Geometry check sheet. Reference: the model listing, model coordinates, mm. A direction names the side the tool comes from. Round coordinates to 2 decimals unless told otherwise and drop trailing zeros. Order: outer loops, then holes, each group sorted by start corner. A loop starts at its lowest first (then second) coordinate and runs counter-clockwise, first axis right, second up.
```python
from build123d import *

# Parameters (mm, degrees)
SKETCH2_W           = 127
SKETCH2_H           = 127
SKETCH2_W_2         = 114.3
SKETCH2_H_2         = 114.3
BOSS_EXTRUDE2_DEPTH = 127
CUT_EXTRUDE1_REACH  = 129
CUT_EXTRUDE2_REACH  = 129


with BuildPart() as part:
    # Sketch2 → Boss-Extrude2 (new body)
    with BuildSketch(Plane(origin=(0, 0, 0), x_dir=(1, 0, 0), z_dir=(0, 1, 0))):
        Rectangle(SKETCH2_W, SKETCH2_H)
        Rectangle(SKETCH2_W_2, SKETCH2_H_2, mode=Mode.SUBTRACT)
    extrude(amount=BOSS_EXTRUDE2_DEPTH)

    # Sketch6 → Cut-Extrude1 (cut, up to next)
    with BuildSketch(Plane.ZY.offset(63.5), mode=Mode.PRIVATE) as cut_extrude1_sk1:
        with BuildLine():
            Line((-4.523172318, 109.1946), (-10.873172318, 109.1946))
            ThreePointArc((-10.873172318, 109.1946), (-13.425872318, 111.7473), (-10.873172318, 114.3))
            Line((-10.873172318, 114.3), (-4.523172318, 114.3))
            ThreePointArc((-4.523172318, 114.3), (-1.970472318, 111.7473), (-4.523172318, 109.1946))
        make_face()
    cut_extrude1_tool1 = extrude(cut_extrude1_sk1.sketch, amount=-CUT_EXTRUDE1_REACH, mode=Mode.PRIVATE) & part.part
    add(cut_extrude1_tool1.solids().sort_by_distance((-63.5, 111.7473, -7.698172))[0], mode=Mode.SUBTRACT)
    # Sketch6 → Cut-Extrude1 (cut, up to next)
    with BuildSketch(Plane.ZY.offset(63.5), mode=Mode.PRIVATE) as cut_extrude1_sk2:
        with BuildLine():
            Line((36.273172318, 114.3), (42.623172318, 114.3))
            ThreePointArc((42.623172318, 114.3), (45.175872318, 111.7473), (42.623172318, 109.1946))
            Line((42.623172318, 109.1946), (36.273172318, 109.1946))
            ThreePointArc((36.273172318, 109.1946), (33.720472318, 111.7473), (36.273172318, 114.3))
        make_face()
    cut_extrude1_tool2 = extrude(cut_extrude1_sk2.sketch, amount=-CUT_EXTRUDE1_REACH, mode=Mode.PRIVATE) & part.part
    add(cut_extrude1_tool2.solids().sort_by_distance((-63.5, 111.7473, 39.448172))[0], mode=Mode.SUBTRACT)
    # Sketch6 → Cut-Extrude1 (cut, up to next)
    with BuildSketch(Plane.ZY.offset(63.5), mode=Mode.PRIVATE) as cut_extrude1_sk3:
        with BuildLine():
            Line((36.273172318, 67.153655364), (42.623172318, 67.153655364))
            ThreePointArc((42.623172318, 67.153655364), (45.175872318, 64.600955364), (42.623172318, 62.048255364))
            Line((42.623172318, 62.048255364), (36.273172318, 62.048255364))
            ThreePointArc((36.273172318, 62.048255364), (33.720472318, 64.600955364), (36.273172318, 67.153655364))
        make_face()
    cut_extrude1_tool3 = extrude(cut_extrude1_sk3.sketch, amount=-CUT_EXTRUDE1_REACH, mode=Mode.PRIVATE) & part.part
    add(cut_extrude1_tool3.solids().sort_by_distance((-63.5, 64.600955, 39.448172))[0], mode=Mode.SUBTRACT)
    # Sketch6 → Cut-Extrude1 (cut, up to next)
    with BuildSketch(Plane.ZY.offset(63.5), mode=Mode.PRIVATE) as cut_extrude1_sk4:
        with BuildLine():
            Line((-4.523172318, 62.048255364), (-10.873172318, 62.048255364))
            ThreePointArc((-10.873172318, 62.048255364), (-13.425872318, 64.600955364), (-10.873172318, 67.153655364))
            Line((-10.873172318, 67.153655364), (-4.523172318, 67.153655364))
            ThreePointArc((-4.523172318, 67.153655364), (-1.970472318, 64.600955364), (-4.523172318, 62.048255364))
        make_face()
    cut_extrude1_tool4 = extrude(cut_extrude1_sk4.sketch, amount=-CUT_EXTRUDE1_REACH, mode=Mode.PRIVATE) & part.part
    add(cut_extrude1_tool4.solids().sort_by_distance((-63.5, 64.600955, -7.698172))[0], mode=Mode.SUBTRACT)
    # Sketch6 → Cut-Extrude1 (cut, up to next)
    with BuildSketch(Plane.ZY.offset(63.5), mode=Mode.PRIVATE) as cut_extrude1_sk5:
        with BuildLine():
            Line((19.05, 83.411627682), (12.7, 83.411627682))
            ThreePointArc((12.7, 83.411627682), (7.9375, 88.174127682), (12.7, 92.936627682))
            Line((12.7, 92.936627682), (19.05, 92.936627682))
            ThreePointArc((19.05, 92.936627682), (23.8125, 88.174127682), (19.05, 83.411627682))
        make_face()
    cut_extrude1_tool5 = extrude(cut_extrude1_sk5.sketch, amount=-CUT_EXTRUDE1_REACH, mode=Mode.PRIVATE) & part.part
    add(cut_extrude1_tool5.solids().sort_by_distance((-63.5, 88.174128, 15.875))[0], mode=Mode.SUBTRACT)

    # Sketch8 → Cut-Extrude2 (cut, up to next)
    with BuildSketch(Plane.XY.offset(63.5), mode=Mode.PRIVATE) as cut_extrude2_sk1:
        with BuildLine():
            Line((-10.250872318, 62.399044636), (-10.250872318, 68.749044636))
            ThreePointArc((-10.250872318, 68.749044636), (-7.698172318, 71.301744636), (-5.145472318, 68.749044636))
            Line((-5.145472318, 68.749044636), (-5.145472318, 62.399044636))
            ThreePointArc((-5.145472318, 62.399044636), (-7.698172318, 59.846344636), (-10.250872318, 62.399044636))
        make_face()
    cut_extrude2_tool1 = extrude(cut_extrude2_sk1.sketch, amount=-CUT_EXTRUDE2_REACH, mode=Mode.PRIVATE) & part.part
    add(cut_extrude2_tool1.solids().sort_by_distance((-7.698172, 65.574045, 63.5))[0], mode=Mode.SUBTRACT)
    # Sketch8 → Cut-Extrude2 (cut, up to next)
    with BuildSketch(Plane.XY.offset(63.5), mode=Mode.PRIVATE) as cut_extrude2_sk2:
        with BuildLine():
            Line((36.895472318, 62.399044636), (36.895472318, 68.749044636))
            ThreePointArc((36.895472318, 68.749044636), (39.448172318, 71.301744636), (42.000872318, 68.749044636))
            Line((42.000872318, 68.749044636), (42.000872318, 62.399044636))
            ThreePointArc((42.000872318, 62.399044636), (39.448172318, 59.846344636), (36.895472318, 62.399044636))
        make_face()
    cut_extrude2_tool2 = extrude(cut_extrude2_sk2.sketch, amount=-CUT_EXTRUDE2_REACH, mode=Mode.PRIVATE) & part.part
    add(cut_extrude2_tool2.solids().sort_by_distance((39.448172, 65.574045, 63.5))[0], mode=Mode.SUBTRACT)
    # Sketch8 → Cut-Extrude2 (cut, up to next)
    with BuildSketch(Plane.XY.offset(63.5), mode=Mode.PRIVATE) as cut_extrude2_sk3:
        with BuildLine():
            Line((42.000872318, 21.6027), (42.000872318, 15.2527))
            ThreePointArc((42.000872318, 15.2527), (39.448172318, 12.7), (36.895472318, 15.2527))
            Line((36.895472318, 15.2527), (36.895472318, 21.6027))
            ThreePointArc((36.895472318, 21.6027), (39.448172318, 24.1554), (42.000872318, 21.6027))
        make_face()
    cut_extrude2_tool3 = extrude(cut_extrude2_sk3.sketch, amount=-CUT_EXTRUDE2_REACH, mode=Mode.PRIVATE) & part.part
    add(cut_extrude2_tool3.solids().sort_by_distance((39.448172, 18.4277, 63.5))[0], mode=Mode.SUBTRACT)
    # Sketch8 → Cut-Extrude2 (cut, up to next)
    with BuildSketch(Plane.XY.offset(63.5), mode=Mode.PRIVATE) as cut_extrude2_sk4:
        with BuildLine():
            Line((-10.250872318, 15.2527), (-10.250872318, 21.6027))
            ThreePointArc((-10.250872318, 21.6027), (-7.698172318, 24.1554), (-5.145472318, 21.6027))
            Line((-5.145472318, 21.6027), (-5.145472318, 15.2527))
            ThreePointArc((-5.145472318, 15.2527), (-7.698172318, 12.7), (-10.250872318, 15.2527))
        make_face()
    cut_extrude2_tool4 = extrude(cut_extrude2_sk4.sketch, amount=-CUT_EXTRUDE2_REACH, mode=Mode.PRIVATE) & part.part
    add(cut_extrude2_tool4.solids().sort_by_distance((-7.698172, 18.4277, 63.5))[0], mode=Mode.SUBTRACT)
    # Sketch8 → Cut-Extrude2 (cut, up to next)
    with BuildSketch(Plane.XY.offset(63.5), mode=Mode.PRIVATE) as cut_extrude2_sk5:
        with BuildLine():
            Line((11.1125, 38.825872318), (11.1125, 45.175872318))
            ThreePointArc((11.1125, 45.175872318), (15.875, 49.938372318), (20.6375, 45.175872318))
            Line((20.6375, 45.175872318), (20.6375, 38.825872318))
            ThreePointArc((20.6375, 38.825872318), (15.875, 34.063372318), (11.1125, 38.825872318))
        make_face()
    cut_extrude2_tool5 = extrude(cut_extrude2_sk5.sketch, amount=-CUT_EXTRUDE2_REACH, mode=Mode.PRIVATE) & part.part
    add(cut_extrude2_tool5.solids().sort_by_distance((15.875, 42.000872, 63.5))[0], mode=Mode.SUBTRACT)


solid = part.part
```
(1) Sectioned sample at A-A, the plane x = -27. Record the cut outline in (y, z).
Returned:
outline: (0, -63.5) - (127, -63.5) - (127, -57.15) - (0, -57.15) - close; (0, 57.15) - (127, 57.15) - (127, 63.5) - (0, 63.5) - close
(2) Material ranges on line 1 (X direction, y = 28, z = -10.5), recorded low to high.
Returned:
line 1: x = -63.5 to -57.15, 57.15 to 63.5
(3) Set-up check for faces 1 (the flat face through (-5.145, 18, 60)), 2 (the cylindrical face through (-60.37, 111.69, 33.72)), 3 (the flat face through (-5, 127, 61)), 4 (the flat face through (57.15, 63, 1)): record each of +Z, -Z, +X, -X, +Y, -Y from which the full face is reachable in a straight line by a thin tool's end or side.
Returned:
face 1: +Z
face 2: -X
face 3: +Z, -Z, +X, -X, +Y
face 4: +Y, -Y
(4) Sectioned sample at B-B, the plane z = -16.5. Record the cut outline in (x, y).
Returned:
outline: (-63.5, 0) - (-57.15, 0) - (-57.15, 127) - (-63.5, 127) - close; (57.15, 0) - (63.5, 0) - (63.5, 127) - (57.15, 127) - close
(5) Sectioned sample at C-C, the plane y = 56.5. Record the cut outline in (x, z).
Returned:
outline: (-63.5, -63.5) - (63.5, -63.5) - (63.5, 63.5) - (-63.5, 63.5) - close; hole (-57.15, -57.15) - (57.15, -57.15) - (57.15, 57.15) - (-57.15, 57.15) - close
(6) Sectioned sample at D-D, the plane z = 15.5. Record the cut outline in (x, y), and give its area (3 significant figures).
Returned:
outline: (-63.5, 0) - (-57.15, 0) - (-57.15, 83.41) - (-63.5, 83.41) - close; (-63.5, 92.94) - (-57.15, 92.94) - (-57.15, 127) - (-63.5, 127) - close; (57.15, 0) - (63.5, 0) - (63.5, 127) - (57.15, 127) - close
area: 1,550 mm2
(7) Draft check along Z on faces 5 (the cylindrical face through (-60.369, 111.803, 45.175)), 6 (the cylindrical face through (-60.37, 64.54, 33.72)), 7 (the flat face through (36.895, 66, 60)). Enter one of: released by +Z, released by -Z, zero draft, split by the parting line, or undercut.
Returned:
face 5: undercut
face 6: undercut
face 7: zero draft
